from build123d import *

# Parameters (mm, degrees)
BOSS_EXTRUDE1_DEPTH = 12.5


with BuildPart() as part:
    # Sketch1 → Boss-Extrude1 (new body)
    with BuildSketch(Plane.XY):
        with BuildLine():
            ThreePointArc((231.15, 12.5), (237.5, 18.85), (243.85, 12.5))
            Line((243.85, 12.5), (250, 12.5))
            Line((250, 12.5), (250, 12.51))
            ThreePointArc((250, 12.51), (246.341763697, 21.341763697), (237.51, 25))
            Line((237.51, 25), (12.49, 25))
            ThreePointArc((12.49, 25), (3.658236303, 21.341763697), (0, 12.51))
            Line((0, 12.51), (0, 12.5))
            Line((0, 12.5), (6.15, 12.5))
            ThreePointArc((6.15, 12.5), (12.5, 18.85), (18.85, 12.5))
            Line((18.85, 12.5), (231.15, 12.5))
        make_face()
        with BuildLine():
            Line((250, 12.5), (243.85, 12.5))
            ThreePointArc((243.85, 12.5), (237.5, 6.15), (231.15, 12.5))
            Line((231.15, 12.5), (18.85, 12.5))
            ThreePointArc((18.85, 12.5), (12.5, 6.15), (6.15, 12.5))
            Line((6.15, 12.5), (0, 12.5))
            Line((0, 12.5), (0, 12.49))
            ThreePointArc((0, 12.49), (3.658236303, 3.658236303), (12.49, 0))
            Line((12.49, 0), (237.51, 0))
            ThreePointArc((237.51, 0), (246.341763697, 3.658236303), (250, 12.49))
            Line((250, 12.49), (250, 12.5))
        make_face()
    extrude(amount=BOSS_EXTRUDE1_DEPTH)


solid = part.part
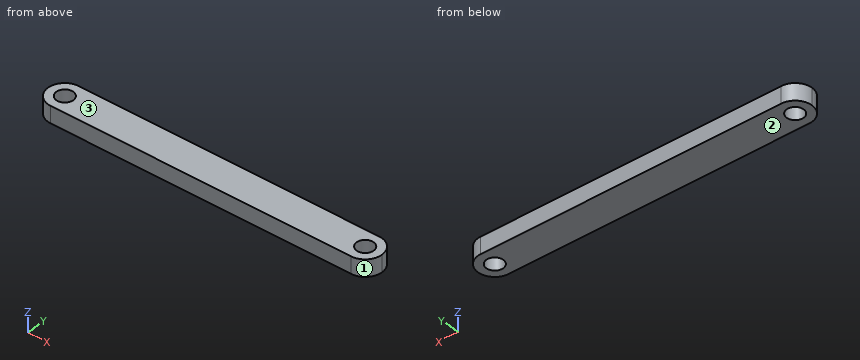
Build history of the part. All positions in model axes, mm. Face numbers are marked on the shaded views. Round coordinates to 2 decimals unless told otherwise and drop trailing zeros. Loops run counter-clockwise (first coordinate to the right, second up) from the corner with the lowest first, then second, coordinate; pieces in that order, holes last. Notation, with made-up numbers: (41.25, 4.5) -> (75.25, 4.5) arc R21 cw to (75.25, 10.5) -> close; hole circle Ø6 at (43.25, 54.5). An arc over 180 degrees is marked (long way). One line per item, written item: value. Start each with the question number.
Q1. Cut at B-B on y = 15. List the corners of the cut face in (x, z), plus the area to 3 significant figures.
Q2. Probe line 1 along X through (y, z) = (12.5, 2.5); line 2 along Y through (x, z) = (12.5, 3.25); line 3 along X through (y, z) = (7.25, 7). List the from-to ranges inside material, lowest first.
Q3. Two-plate mould, pull along Z, no slides. Class the marked faces 1, 2 and 3: released by +Z, released by -Z, zero draft, split by the parting line, or undercut.
Q4. Drop flat-ended pins along their axis: pin 1 Ø3 at (y, z) = (7, 8.5) entering from +X; pin 2 Ø4 at (y, z) = (9.5, 3) entering from -X; pin 3 Ø3 at (y, z) = (20.5, 3.5) entering from +X. Give the stop position or say it passes through.
Q5. Cut at A-A on z = 7.5. Count the separate pieces of the cut face and the enclosed holes in it, plus the area to 3 significant figures.
Q6. Cut at C-C on y = 2.5. List the corners of the cut face in (x, z).
Computed:
1. outline: (0.25, 0) -> (6.66, 0) -> (6.66, 12.5) -> (0.25, 12.5) -> close; (18.34, 0) -> (231.66, 0) -> (231.66, 12.5) -> (18.34, 12.5) -> close; (243.34, 0) -> (249.75, 0) -> (249.75, 12.5) -> (243.34, 12.5) -> close
1. area: 2,830 mm²
2. line 1: 0 to 6.15, 18.85 to 231.15, 243.85 to 250
2. line 2: 0 to 6.15, 18.85 to 25
2. line 3: 1.15 to 8.93, 16.07 to 233.93, 241.07 to 248.85
3. face 1: zero draft
3. face 2: released by -Z
3. face 3: released by +Z
4. pin 1: x = 249.35
4. pin 2: x = 0.04
4. pin 3: x = 248.18
5. separate pieces: 1
5. enclosed holes: 2
5. area: 5,860 mm²
6. outline: (4.99, 0) -> (245.01, 0) -> (245.01, 12.5) -> (4.99, 12.5) -> close
